The model under review builds one solid part; all positions refer to its coordinate system, in mm. A direction names the side the tool comes from. Coordinates: 2 decimals unless noted, no trailing zeros. Loops run counter-clockwise (first coordinate to the right, second up) from the corner with the lowest first, then second, coordinate; pieces in that order, holes last. Notation, with made-up numbers: M 43,52.25 L 65,52.25 A34 ccw 65,84.25 Z; hole C 67,53.5 d9. An arc over 180 degrees is marked long. Return JSON: item names as keys, results as strings.
```python
from build123d import *

# Parameters (mm, degrees)
SKETCH_R     = 7.5
PAD_DEPTH    = 24
SKETCH001_R  = 1.5
PAD001_DEPTH = 3
SKETCH002_R  = 1.5
PAD002_DEPTH = 4
SKETCH003_R  = 4
PAD003_DEPTH = 2
SKETCH004_R  = 2.5
PAD004_DEPTH = 2
SKETCH005_R  = 4
PAD005_DEPTH = 2


with BuildPart() as part:
    # Sketch → Pad (new body)
    with BuildSketch(Plane.XY):
        Circle(SKETCH_R)
    extrude(amount=PAD_DEPTH)

    # Sketch001 → Pad001 (new body)
    with BuildSketch(Plane.XY.offset(24)):
        Circle(SKETCH001_R)
    extrude(amount=PAD001_DEPTH)

    # Sketch002 → Pad002 (new body)
    with BuildSketch(Plane(origin=(0, 0, 0), x_dir=(1, 0, 0), z_dir=(0, 0, -1))):
        Circle(SKETCH002_R)
    extrude(amount=PAD002_DEPTH)

    # Sketch003 → Pad003 (new body)
    with BuildSketch(Plane(origin=(0, 0, -4), x_dir=(1, 0, 0), z_dir=(0, 0, -1))):
        Circle(SKETCH003_R)
    extrude(amount=PAD003_DEPTH)

    # Sketch004 → Pad004 (new body)
    with BuildSketch(Plane(origin=(0, 0, -6), x_dir=(1, 0, 0), z_dir=(0, 0, -1))):
        Circle(SKETCH004_R)
    extrude(amount=PAD004_DEPTH)

    # Sketch005 → Pad005 (new body)
    with BuildSketch(Plane(origin=(0, 0, -8), x_dir=(1, 0, 0), z_dir=(0, 0, -1))):
        Circle(SKETCH005_R)
    extrude(amount=PAD005_DEPTH)


solid = part.part
```
1. To check wall thickness, follow line 1 (Z direction, x = -0.5, y = 1.75); line 2 (Z direction, x = 1.75, y = -3.5); line 3 (Z direction, x = -4, y = 4.75). State the ranges of each line that lie inside material, in increasing order.
Check values:
{"line 1": "-10 to -4, 0 to 24", "line 2": "-10 to -8, -6 to -4, 0 to 24", "line 3": "0 to 24"}
2. Add section C-C on y = 0. Give the boundary of the cut face in (x, z), plus the area to 3 significant figures.
Check values:
{"outline": "M -7.5,0 L -1.5,0 L -1.5,-4 L -4,-4 L -4,-6 L -2.5,-6 L -2.5,-8 L -4,-8 L -4,-10 L 4,-10 L 4,-8 L 2.5,-8 L 2.5,-6 L 4,-6 L 4,-4 L 1.5,-4 L 1.5,0 L 7.5,0 L 7.5,24 L 1.5,24 L 1.5,27 L -1.5,27 L -1.5,24 L -7.5,24 Z", "area": "423 mm²"}
3. Insertion check: pin 1 Ø7.5 at (x, y) = (-3.5, 0.5) entering from +Z; pin 2 Ø3 at (y, z) = (-3, 10.5) entering from -X; pin 3 Ø2 at (y, z) = (3, 2) entering from +X; pin 4 Ø4 at (x, y) = (1, -3.5) entering from +Z. Each pin has a flat end and moves straight along its axis. Give the tip position at first contact, or say it passes through.
Check values:
{"pin 1": "z = 27", "pin 2": "x = -7.35", "pin 3": "x = 7.23", "pin 4": "z = 24"}
4. Add section D-D on z = 20.5. Give the boundary of the cut face in (x, y), plus the area to 3 significant figures.
Check values:
{"outline": "C 0,0 d15", "area": "177 mm²"}
5. Machinability: for faces 1 (the face through (-0.54, 2.44, -6.99)), 2 (the face through (-1.5, 0.07, 25.48)), 3 (the face through (-0.867, 3.905, -4.986)), which of the approach directions +Z, -Z, +X, -X, +Y, -Y give a long, thin tool a straight path to every point of the face, cutting with its end or side? Answer none if there is none.
Check values:
{"face 1": "none", "face 2": "+Z", "face 3": "-Z"}
6. Add section B-B on x = 0.75. Give the boundary of the cut face in (y, z), plus the area to 3 significant figures.
Check values:
{"outline": "M -7.46,0 L -1.3,0 L -1.3,-4 L -3.93,-4 L -3.93,-6 L -2.38,-6 L -2.38,-8 L -3.93,-8 L -3.93,-10 L 3.93,-10 L 3.93,-8 L 2.38,-8 L 2.38,-6 L 3.93,-6 L 3.93,-4 L 1.3,-4 L 1.3,0 L 7.46,0 L 7.46,24 L 1.3,24 L 1.3,27 L -1.3,27 L -1.3,24 L -7.46,24 Z", "area": "417 mm²"}
7. The part is to be moulded in two halves that separate along Z. For faces 4 (the face through (-7.493, 0.33, 11.832)), 5 (the face through (2, 0, -4)), 6 (the face through (0, 0, -10)), say which applies: released by +Z, released by -Z, zero draft, split by the parting line, or undercut.
Check values:
{"face 4": "zero draft", "face 5": "undercut", "face 6": "released by -Z"}
8. Add section A-A on y = -3.5. Give the boundary of the cut face in (x, z), plus the area to 3 significant figures.
Check values:
{"outline": "M -6.63,0 L 6.63,0 L 6.63,24 L -6.63,24 Z; M -1.94,-10 L 1.94,-10 L 1.94,-8 L -1.94,-8 Z; M -1.94,-6 L 1.94,-6 L 1.94,-4 L -1.94,-4 Z", "area": "334 mm²"}
